from build123d import *

# Parameters (mm, degrees)
ESBO_O1_W                = 89.1
ESBO_O1_H                = 70
ESBO_O1_W_2              = 51.55
ESBO_O1_H_2              = 69
ESBO_O1_W_3              = 35.55
RESSALTO_EXTRUS_O1_DEPTH = 150
ESBO_O3_R                = 2
ESBO_O3_R_2              = 4.5
CORTE_EXTRUS_O1_DEPTH    = 1


with BuildPart() as part:
    # Esboço1 → Ressalto-extrusão1 (new body)
    with BuildSketch(Plane(origin=(0, 0, 0), x_dir=(1, 0, 0), z_dir=(0, 1, 0))):
        Rectangle(ESBO_O1_W, ESBO_O1_H)
        with Locations((18.275, 0)):
            Rectangle(ESBO_O1_W_2, ESBO_O1_H_2, mode=Mode.SUBTRACT)
        with Locations((-26.275, 0)):
            Rectangle(ESBO_O1_W_3, ESBO_O1_H_2, mode=Mode.SUBTRACT)
    extrude(amount=RESSALTO_EXTRUS_O1_DEPTH)

    # Esboço3 → Corte-extrusão1 (cut)
    with BuildSketch(Plane(origin=(-7.5, 0, 0), x_dir=(0, 0, -1), z_dir=(1, 0, 0))):
        with Locations((17.5, 75.034551114)):
            Circle(ESBO_O3_R)
        with Locations((-17.5, 75.034551114)):
            Circle(ESBO_O3_R)
        with Locations((0, 83.034551114)):
            Circle(ESBO_O3_R_2)
    extrude(amount=-CORTE_EXTRUS_O1_DEPTH, mode=Mode.SUBTRACT)


solid = part.part
Model file for the job. Use its own axes, mm. A direction names the side the tool comes from. Give positions to 0.01 mm unless a question says otherwise; leave off trailing zeros. Order: outer loops, then holes, each group sorted by start corner. A loop starts at its lowest first (then second) coordinate and runs counter-clockwise, first axis right, second up. Notation, with made-up numbers: (-6.75, 21.25) - (46.25, 21.25) arc R21 cw to (46.25, 59.25) - close; hole circle Ø8 at (-28, 55.25). An arc over 180 degrees is marked (long way). Write item = value, one per line. Start each with the question number.
1. Two-plate mould, pull along Y, no slides. Class faces 4 (the cylindrical face through (-7.99, 73.08, -17.07)), 5 (the flat face through (18, 74, -34.5)), 6 (the cylindrical face through (-7.993, 79.042, -2.076)): pulls with the +Y half, pulls with the -Y half, needs draft (parallel to the pull), parting line crosses it, or undercut.
2. Cut at D-D, the plane z = -23. List the corners of the cut face in (x, y).
3. Cut at B-B, the plane x = -15. List the corners of the cut face in (y, z).
4. Which spindle directions (+Z, -Z, +X, -X, +Y, -Y) get a long thin tool onto all of the face, cutting with end or side? Do faces 1 (the cylindrical face through (-7.99, 73.08, 17.93)), 2 (the flat face through (-44.05, 74, 0)), 3 (the flat face through (-44.55, 74, 0)). Say none if no direction does.
5. Cut at C-C, the plane y = 62. List the corners of the cut face in (x, z), and give its area (3 significant figures).
6. Probe line 1 along X through (y, z) = (66, 22); line 2 along Z through (x, y) = (29.5, 76.5); line 3 along X through (y, z) = (75.5, 16.5). List the from-to ranges inside material, lowest first.
7. Cut at A-A, the plane z = 0. List the corners of the cut face in (x, y), and give its area (3 significant figures).
Taken from the geometry:
q1.face_4 = undercut
q1.face_5 = needs draft
q1.face_6 = undercut
q2.outline = (-44.55, 0) - (-44.05, 0) - (-44.05, 150) - (-44.55, 150) - close; (-8.5, 0) - (-7.5, 0) - (-7.5, 150) - (-8.5, 150) - close; (44.05, 0) - (44.55, 0) - (44.55, 150) - (44.05, 150) - close
q3.outline = (0, -35) - (150, -35) - (150, -34.5) - (0, -34.5) - close; (0, 34.5) - (150, 34.5) - (150, 35) - (0, 35) - close
q4.face_1 = none
q4.face_2 = +Y, -Y
q4.face_3 = +Z, -Z, -X, +Y, -Y
q5.outline = (-44.55, -35) - (44.55, -35) - (44.55, 35) - (-44.55, 35) - close; hole (-44.05, -34.5) - (-8.5, -34.5) - (-8.5, 34.5) - (-44.05, 34.5) - close; hole (-7.5, -34.5) - (44.05, -34.5) - (44.05, 34.5) - (-7.5, 34.5) - close
q5.area = 227 mm²
q6.line_1 = -44.55 to -44.05, -8.5 to -7.5, 44.05 to 44.55
q6.line_2 = -35 to -34.5, 34.5 to 35
q6.line_3 = -44.55 to -44.05, 44.05 to 44.55
q7.outline = (-44.55, 0) - (-44.05, 0) - (-44.05, 150) - (-44.55, 150) - close; (-8.5, 0) - (-7.5, 0) - (-7.5, 78.53) - (-8.5, 78.53) - close; (-8.5, 87.53) - (-7.5, 87.53) - (-7.5, 150) - (-8.5, 150) - close; (44.05, 0) - (44.55, 0) - (44.55, 150) - (44.05, 150) - close
q7.area = 291 mm²
